The listing builds one solid part. Answer for the finished solid, in the listing's coordinates (mm). A direction names the side the tool comes from. Coordinates: 2 decimals unless noted, no trailing zeros. Order: outer loops, then holes, each group sorted by start corner. A loop starts at its lowest first (then second) coordinate and runs counter-clockwise, first axis right, second up. Notation, with made-up numbers: (41, -40) -> (93, -40) arc R18 cw to (93, -32) -> close; hole circle Ø1 at (69, 14). An arc over 180 degrees is marked (long way). Answer in a Markdown table with one row per item.
```python
from build123d import *

# Parameters (mm, degrees)
F1_DEPTH = 25.4
F2_R     = 6.35
F3_DEPTH = 25.4
F5_DEPTH = 12.7


with BuildPart() as f1:
    # F0 (on Front) → F1 (new body)
    with BuildSketch(Plane.XZ):
        Polygon((0, 38.1), (0, 0), (69.85, 0), (69.85, 12.7), (25.4, 12.7), (25.4, 38.1), align=None)
    extrude(amount=F1_DEPTH)

    # F2 (on face) → F3 (cut)
    with BuildSketch(Plane.XZ.offset(25.4)):
        with Locations((12.7, 25.4)):
            Circle(F2_R)
        with BuildLine():
            ThreePointArc((12.7, 38.1), (21.680256, 34.380256), (25.4, 25.4))
            Line((25.4, 25.4), (25.4, 38.1))
            Line((25.4, 38.1), (12.7, 38.1))
        make_face()
        with BuildLine():
            ThreePointArc((0, 25.4), (3.719744, 34.380256), (12.7, 38.1))
            Line((12.7, 38.1), (0, 38.1))
            Line((0, 38.1), (0, 25.4))
        make_face()
    extrude(amount=-F3_DEPTH, mode=Mode.SUBTRACT)

    # F4 (on face) → F5 (cut)
    with BuildSketch(Plane.XY.offset(12.7)):
        with BuildLine():
            ThreePointArc((44.918065, -12.7), (43.058193, -8.209872), (38.568065, -6.35))
            ThreePointArc((38.568065, -6.35), (32.218065, -12.7), (38.568065, -19.05))
            ThreePointArc((38.568065, -19.05), (43.058193, -17.190128), (44.918065, -12.7))
        make_face()
        with BuildLine():
            ThreePointArc((56.72131, -19.05), (50.37131, -12.7), (56.72131, -6.35))
            Line((56.72131, -6.35), (38.568065, -6.35))
            ThreePointArc((38.568065, -6.35), (43.058193, -8.209872), (44.918065, -12.7))
            ThreePointArc((44.918065, -12.7), (43.058193, -17.190128), (38.568065, -19.05))
            Line((38.568065, -19.05), (56.72131, -19.05))
        make_face()
        with BuildLine():
            ThreePointArc((56.72131, -19.05), (61.211438, -17.190128), (63.07131, -12.7))
            ThreePointArc((63.07131, -12.7), (61.211438, -8.209872), (56.72131, -6.35))
            ThreePointArc((56.72131, -6.35), (50.37131, -12.7), (56.72131, -19.05))
        make_face()
        with BuildLine():
            ThreePointArc((56.72131, 0), (69.42131, -12.7), (56.72131, -25.4))
            Line((56.72131, -25.4), (69.85, -25.4))
            Line((69.85, -25.4), (69.85, 0))
            Line((69.85, 0), (56.72131, 0))
        make_face()
    extrude(amount=-F5_DEPTH, mode=Mode.SUBTRACT)


solid = f1.part
```
(1) A cutting plane is placed at A-A, the plane y = -9.5. Determine the outline of the cut face in (x, z), then the cut area to 3 significant figures.
Check values:
| item | result |
|---|---|
| outline | (0, 0) -> (33.08, 0) -> (33.08, 12.7) -> (25.4, 12.7) -> (25.4, 25.4) arc R12.7 ccw to (0, 25.4) -> close; (62.21, 0) -> (69.01, 0) -> (69.01, 12.7) -> (62.21, 12.7) -> close; hole circle Ø12.7 at (12.7, 25.4) |
| area | 956 mm² |
(2) Find the intervals of material crossed by line 1 along Z through (x, y) = (12.7, -15.5); line 2 along X through (y, z) = (-2.5, 19); line 3 along Z through (x, y) = (62.5, -5), in increasing order. Write a range as from..to.
Check values:
| item | result |
|---|---|
| line 1 | 0..19.05, 31.75..38.1 |
| line 2 | 0..25.4 |
| line 3 | 0..12.7 |
(3) A cutting plane is placed at D-D, the plane z = 21. Determine the outline of the cut face in (x, y), then the cut area to 3 significant figures.
Check values:
| item | result |
|---|---|
| outline | (0, -25.4) -> (8.12, -25.4) -> (8.12, 0) -> (0, 0) -> close; (17.28, -25.4) -> (25.4, -25.4) -> (25.4, 0) -> (17.28, 0) -> close |
| area | 413 mm² |
(4) Flat-ended cylindrical pins translate along their axes: pin 1 (3 mm diameter, centred on y = -3.5, z = 33.5, fed in from +X); pin 2 (5 mm diameter, centred on x = 33.5, y = -7, fed in from +Z); pin 3 (14 mm diameter, centred on y = -14, z = 22, fed in from +X). Find the tip coordinate at first contact, or state that the pin passes through.
Check values:
| item | result |
|---|---|
| pin 1 | x = 23.55 |
| pin 2 | z = 12.7 |
| pin 3 | x = 25.4 |
(5) A cutting plane is placed at B-B, the plane z = 6.5. Determine the outline of the cut face in (x, y).
Check values:
| item | result |
|---|---|
| outline | (0, -25.4) -> (56.72, -25.4) arc R12.7 ccw to (56.72, 0) -> (0, 0) -> close; hole (38.57, -19.05) -> (56.72, -19.05) arc R6.35 ccw to (56.72, -6.35) -> (38.57, -6.35) arc R6.35 ccw to start |
(6) For a pull along X with two mould halves and no side action, classify faces 1 (the flat face through (27, -13, 0)), 2 (the cylindrical face through (69.42, -12.42, 6.44)), 3 (the cylindrical face through (7.66, -12.88, 21.54)) as released by +X, released by -X, zero draft, split by the parting line, or undercut.
Check values:
| item | result |
|---|---|
| face 1 | zero draft |
| face 2 | released by +X |
| face 3 | undercut |
(7) Which of the six approach directions +Z, -Z, +X, -X, +Y, -Y give full straight-line access (tool end or side, diameter ignored) to faces 4 (the flat face through (22, 0, 15)), 5 (the flat face through (25.4, -13, 19)), 6 (the flat face through (48, -6.35, 6))?
Check values:
| item | result |
|---|---|
| face 4 | +Z, -Z, +X, -X, +Y |
| face 5 | +Z, +X, +Y, -Y |
| face 6 | +Z, -Z |
(8) A cutting plane is placed at C-C, the plane x = 49. Determine the outline of the cut face in (y, z).
Check values:
| item | result |
|---|---|
| outline | (-25.4, 0) -> (-19.05, 0) -> (-19.05, 12.7) -> (-25.4, 12.7) -> close; (-6.35, 0) -> (0, 0) -> (0, 12.7) -> (-6.35, 12.7) -> close |
